The model under review builds one solid part; all positions refer to its coordinate system, in mm. A direction names the side the tool comes from. Coordinates: 2 decimals unless noted, no trailing zeros. Write each loop counter-clockwise with the first axis right and the second up, starting at its lowest first coordinate (ties: lowest second). Pieces come first, ordered by that corner, then holes.
```python
from build123d import *

# Parameters (mm, degrees)
F0_W     = 76.52381
F0_H     = 52.565604
F1_DEPTH = 25.4
F3_DEPTH = 25.4


with BuildPart() as f1:
    # F0 (on Top) → F1 (new body)
    with BuildSketch(Plane.XY):
        Rectangle(F0_W, F0_H)
    extrude(amount=F1_DEPTH)

    # F2 (on face) → F3 (join)
    with BuildSketch(Plane.XY.offset(25.4)):
        with BuildLine():
            Line((38.261905, 26.282802), (14.039008, 26.282802))
            ThreePointArc((14.039008, 26.282802), (2.519291, 0), (14.039008, -26.282802))
            Line((14.039008, -26.282802), (38.261905, -26.282802))
            Line((38.261905, -26.282802), (38.261905, 26.282802))
        make_face()
    extrude(amount=F3_DEPTH)


solid = f1.part
```
Item 1: For pin 1 (8 mm diameter, centred on x = -13.5, y = 4, fed in from +Z); pin 2 (3 mm diameter, centred on x = 4, z = 30, fed in from +Y); pin 3 (1 mm diameter, centred on y = 14.5, z = 36.5, fed in from -X); pin 4 (10 mm diameter, centred on x = -17.5, z = 34, fed in from +Y), all flat-tipped, find the tip position at first contact; note any pin that passes through.
Solved:
pin 1: stops at z = 25.4
pin 2: stops at y = 14.29
pin 3: stops at x = 5.38
pin 4: passes through
Item 2: To check wall thickness, follow line 1 along Z through (x, y) = (-10.5, -14); line 2 along X through (y, z) = (-17, 35.5); line 3 along X through (y, z) = (12, 46.5). State the ranges of each line that lie inside material, in increasing order.
Solved:
line 1: z = 0 to 25.4
line 2: x = 6.82 to 38.26
line 3: x = 4.59 to 38.26
Item 3: Take a section at B-B, the plane y = 9.5. Write out the cut boundary in (x, z).
Solved:
outline: (-38.26, 0) - (38.26, 0) - (38.26, 50.8) - (3.8, 50.8) - (3.8, 25.4) - (-38.26, 25.4) - close
Item 4: Take a section at D-D, the plane y = -5.5. Write out the cut boundary in (x, z) (3 decimals), plus the area to 3 significant figures.
Solved:
outline: (-38.262, 0) - (38.262, 0) - (38.262, 50.8) - (2.945, 50.8) - (2.945, 25.4) - (-38.262, 25.4) - close
area: 2,840 mm2
Item 5: Take a section at C-C, the plane x = 7. Write out the cut boundary in (y, z).
Solved:
outline: (-26.28, 0) - (26.28, 0) - (26.28, 25.4) - (17.33, 25.4) - (17.33, 50.8) - (-17.33, 50.8) - (-17.33, 25.4) - (-26.28, 25.4) - close
Item 6: Machinability: for faces 1 (the face through (20, 0, 50.8)), 2 (the face through (2.52, 0.41, 37.92)), which of the approach directions +Z, -Z, +X, -X, +Y, -Y give a long, thin tool a straight path to every point of the face, cutting with its end or side? Answer none if there is none.
Solved:
face 1: +Z, +X, -X, +Y, -Y
face 2: +Z, -X
Item 7: Take a section at A-A, the plane z = 38. Write out the cut boundary in (x, y), plus the area to 3 significant figures.
Solved:
outline: (14.04, -26.28) - (38.26, -26.28) - (38.26, 26.28) - (14.04, 26.28) arc R35.74 ccw to start
area: 1,690 mm2
